from build123d import *

# Parameters (mm, degrees)
SKETCH1_W           = 55
SKETCH1_H           = 39
BOSS_EXTRUDE1_DEPTH = 1
CUT_EXTRUDE1_REACH  = 69.431
SKETCH3_R           = 1
SKETCH3_R_2         = 4.5
SKETCH2_W           = 7
SKETCH2_H           = 10
BOSS_EXTRUDE2_DEPTH = 24.1
CUT_EXTRUDE2_REACH  = 67.81
SKETCH4_R           = 1


with BuildPart() as part:
    # Sketch1 → Boss-Extrude1 (new body)
    with BuildSketch(Plane(origin=(0, 0, 0), x_dir=(1, 0, 0), z_dir=(0, 1, 0))):
        with Locations((27.5, 19.5)):
            Rectangle(SKETCH1_W, SKETCH1_H)
    extrude(amount=BOSS_EXTRUDE1_DEPTH)

    # Sketch3 → Cut-Extrude1 (cut, up to next)
    with BuildSketch(Plane(origin=(0, 1, 0), x_dir=(1, 0, 0), z_dir=(0, 1, 0)), mode=Mode.PRIVATE) as cut_extrude1_sk1:
        with Locations(Location((34.5, 26.5, 0), (0, 0, 270))):
            Circle(SKETCH3_R)
    cut_extrude1_tool1 = extrude(cut_extrude1_sk1.sketch, amount=-CUT_EXTRUDE1_REACH, mode=Mode.PRIVATE) & part.part
    # Sketch3 → Cut-Extrude1 (cut, up to next)
    with BuildSketch(Plane(origin=(0, 1, 0), x_dir=(1, 0, 0), z_dir=(0, 1, 0)), mode=Mode.PRIVATE) as cut_extrude1_sk2:
        with Locations(Location((34.5, 12.5, 0), (0, 0, 270))):
            Circle(SKETCH3_R)
    cut_extrude1_tool2 = extrude(cut_extrude1_sk2.sketch, amount=-CUT_EXTRUDE1_REACH, mode=Mode.PRIVATE) & part.part
    # Sketch3 → Cut-Extrude1 (cut, up to next)
    with BuildSketch(Plane(origin=(0, 1, 0), x_dir=(1, 0, 0), z_dir=(0, 1, 0)), mode=Mode.PRIVATE) as cut_extrude1_sk3:
        with Locations(Location((20.5, 12.5, 0), (0, 0, 270))):
            Circle(SKETCH3_R)
    cut_extrude1_tool3 = extrude(cut_extrude1_sk3.sketch, amount=-CUT_EXTRUDE1_REACH, mode=Mode.PRIVATE) & part.part
    # Sketch3 → Cut-Extrude1 (cut, up to next)
    with BuildSketch(Plane(origin=(0, 1, 0), x_dir=(1, 0, 0), z_dir=(0, 1, 0)), mode=Mode.PRIVATE) as cut_extrude1_sk4:
        with Locations(Location((20.5, 26.5, 0), (0, 0, 270))):
            Circle(SKETCH3_R)
    cut_extrude1_tool4 = extrude(cut_extrude1_sk4.sketch, amount=-CUT_EXTRUDE1_REACH, mode=Mode.PRIVATE) & part.part
    # Sketch3 → Cut-Extrude1 (cut, up to next)
    with BuildSketch(Plane(origin=(0, 1, 0), x_dir=(1, 0, 0), z_dir=(0, 1, 0)), mode=Mode.PRIVATE) as cut_extrude1_sk5:
        with Locations(Location((27.5, 19.5, 0), (0, 0, 270))):
            Circle(SKETCH3_R_2)
    cut_extrude1_tool5 = extrude(cut_extrude1_sk5.sketch, amount=-CUT_EXTRUDE1_REACH, mode=Mode.PRIVATE) & part.part
    add(cut_extrude1_tool1.solids().sort_by_distance((34.5, 1, -26.5))[0], mode=Mode.SUBTRACT)
    add(cut_extrude1_tool2.solids().sort_by_distance((34.5, 1, -12.5))[0], mode=Mode.SUBTRACT)
    add(cut_extrude1_tool3.solids().sort_by_distance((20.5, 1, -12.5))[0], mode=Mode.SUBTRACT)
    add(cut_extrude1_tool4.solids().sort_by_distance((20.5, 1, -26.5))[0], mode=Mode.SUBTRACT)
    add(cut_extrude1_tool5.solids().sort_by_distance((27.5, 1, -19.5))[0], mode=Mode.SUBTRACT)

    # Sketch2 → Boss-Extrude2 (add)
    with BuildSketch(Plane(origin=(0, 1, 0), x_dir=(1, 0, 0), z_dir=(0, 1, 0))):
        with Locations((51.5, 18)):
            Rectangle(SKETCH2_W, SKETCH2_H)
        with Locations((3.5, 18)):
            Rectangle(SKETCH2_W, SKETCH2_H)
    extrude(amount=BOSS_EXTRUDE2_DEPTH)

    # Sketch4 → Cut-Extrude2 (cut, up to next)
    with BuildSketch(Plane.XY.offset(-13), mode=Mode.PRIVATE) as cut_extrude2_sk1:
        with Locations((2.5, 17.95)):
            Circle(SKETCH4_R)
    cut_extrude2_tool1 = extrude(cut_extrude2_sk1.sketch, amount=-CUT_EXTRUDE2_REACH, mode=Mode.PRIVATE) & part.part
    # Sketch4 → Cut-Extrude2 (cut, up to next)
    with BuildSketch(Plane.XY.offset(-13), mode=Mode.PRIVATE) as cut_extrude2_sk2:
        with Locations((2.5, 8.35)):
            Circle(SKETCH4_R)
    cut_extrude2_tool2 = extrude(cut_extrude2_sk2.sketch, amount=-CUT_EXTRUDE2_REACH, mode=Mode.PRIVATE) & part.part
    # Sketch4 → Cut-Extrude2 (cut, up to next)
    with BuildSketch(Plane.XY.offset(-13), mode=Mode.PRIVATE) as cut_extrude2_sk3:
        with Locations((52.5, 8.35)):
            Circle(SKETCH4_R)
    cut_extrude2_tool3 = extrude(cut_extrude2_sk3.sketch, amount=-CUT_EXTRUDE2_REACH, mode=Mode.PRIVATE) & part.part
    # Sketch4 → Cut-Extrude2 (cut, up to next)
    with BuildSketch(Plane.XY.offset(-13), mode=Mode.PRIVATE) as cut_extrude2_sk4:
        with Locations((52.5, 17.95)):
            Circle(SKETCH4_R)
    cut_extrude2_tool4 = extrude(cut_extrude2_sk4.sketch, amount=-CUT_EXTRUDE2_REACH, mode=Mode.PRIVATE) & part.part
    add(cut_extrude2_tool1.solids().sort_by_distance((2.5, 17.95, -13))[0], mode=Mode.SUBTRACT)
    add(cut_extrude2_tool2.solids().sort_by_distance((2.5, 8.35, -13))[0], mode=Mode.SUBTRACT)
    add(cut_extrude2_tool3.solids().sort_by_distance((52.5, 8.35, -13))[0], mode=Mode.SUBTRACT)
    add(cut_extrude2_tool4.solids().sort_by_distance((52.5, 17.95, -13))[0], mode=Mode.SUBTRACT)


solid = part.part
Could you check a few things on this model? Use its own coordinates, in mm. A direction names the side the tool comes from. Give positions to 0.01 mm unless a question says otherwise; leave off trailing zeros. Order: outer loops, then holes, each group sorted by start corner. A loop starts at its lowest first (then second) coordinate and runs counter-clockwise, first axis right, second up. Notation, with made-up numbers: (85.5, 50.25) - (141.5, 50.25) arc R14 cw to (141.5, 66.25) - close; hole circle Ø10 at (23.5, 14). An arc over 180 degrees is marked (long way). One line per item, written item: value. Start each with the question number.
1. Imagine slicing it at B-B on x = 52.5. List the corners of the cut face in (y, z) for me.
2. If I drill on probe 1 along X at (y, z) = (18, -16); probe 2 along X at (y, z) = (0.8, -12.5); probe 3 along Y at (x, z) = (2.5, -18), over which ranges is the centre line in solid material (lowest first)?
3. Imagine slicing it at D-D on x = 27.5. List the corners of the cut face in (y, z) for me, plus the area to 3 significant figures.
4. Thinking about a two-plate mould opening in Y: for faces 6 (the face through (51, 25.1, -18)), 7 (the face through (52.283, 7.374, -17.93)), 8 (the face through (7, 13, -18)), which applies, +Y half, -Y half, draft (parallel to the pull), parting line (faces both ways), or undercut?
5. For P1, Ø4, axis at x = 43, z = -5.5, coming from the -Y side; P2, Ø2.5, axis at x = 2.5, y = 17.95, coming from the -Z side; P3, Ø7.5, axis at x = 2, y = 16, coming from the +Z side; P4, Ø12, axis at y = 21, z = -33, coming from the -X side, each with a flat end and sliding along its axis, tell me the tip position at first contact or that it passes through.
6. For faces 1 (the face through (51, 13, -23)), 2 (the face through (0, 11, -18)), 3 (the face through (48, 13, -18)), 4 (the face through (1.71, 7.74, -17.93)), 5 (the face through (3, 13, -13)), which set-ups out of +Z, -Z, +X, -X, +Y, -Y let a thin tool reach every point of the face, with its end or its side?
7. Imagine slicing it at C-C on y = 17.95. List the corners of the cut face in (x, z) for me.
8. Imagine slicing it at A-A on z = -19.5. List the corners of the cut face in (x, y) for me.
Values:
1. outline: (0, -39) - (1, -39) - (1, -23) - (7.35, -23) - (7.35, -13) - (1, -13) - (1, 0) - (0, 0) - close; (9.35, -23) - (16.95, -23) - (16.95, -13) - (9.35, -13) - close; (18.95, -23) - (25.1, -23) - (25.1, -13) - (18.95, -13) - close
2. probe 1: 0 to 1.5, 3.5 to 7, 48 to 51.5, 53.5 to 55
2. probe 2: 0 to 19.5, 21.5 to 33.5, 35.5 to 55
2. probe 3: 0 to 7.35, 9.35 to 16.95, 18.95 to 25.1
3. outline: (0, -39) - (1, -39) - (1, -24) - (0, -24) - close; (0, -15) - (1, -15) - (1, 0) - (0, 0) - close
3. area: 30.0 mm²
4. face 6: +Y half
4. face 7: undercut
4. face 8: draft
5. P1: y = 0
5. P2: z = -23
5. P3: z = -13
5. P4: through
6. face 1: -Z, +X, -X, +Y
6. face 2: +Z, -Z, -X, +Y, -Y
6. face 3: +Z, -Z, +Y
6. face 4: +Z, -Z
6. face 5: +Z, +X, -X, +Y
7. outline: (0, -23) - (1.5, -23) - (1.5, -13) - (0, -13) - close; (3.5, -23) - (7, -23) - (7, -13) - (3.5, -13) - close; (48, -23) - (51.5, -23) - (51.5, -13) - (48, -13) - close; (53.5, -23) - (55, -23) - (55, -13) - (53.5, -13) - close
8. outline: (0, 0) - (23, 0) - (23, 1) - (7, 1) - (7, 25.1) - (0, 25.1) - close; (32, 0) - (55, 0) - (55, 25.1) - (48, 25.1) - (48, 1) - (32, 1) - close; hole circle Ø2 at (2.5, 8.35); hole circle Ø2 at (2.5, 17.95); hole circle Ø2 at (52.5, 8.35); hole circle Ø2 at (52.5, 17.95)
